Model file for the job. Use its own axes, mm. Coordinates: 2 decimals unless noted, no trailing zeros. Loops run counter-clockwise (first coordinate to the right, second up) from the corner with the lowest first, then second, coordinate; pieces in that order, holes last. Notation, with made-up numbers: M -24,70.5 L 34,70.5 A30 ccw 34,101.5 Z; hole C 45,71.5 d11. An arc over 180 degrees is marked long. One line per question, with ' | ' between items. Start each with the question number.
Autodesk Inventor part; units mm, degrees
ref_plane "YZ Plane" through (0, 0, 0) normal (1, 0, 0) x (0, 1, 0)
ref_plane "XZ Plane" through (0, 0, 0) normal (0, 1, 0) x (-1, 0, 0)
ref_plane "XY Plane" through (0, 0, 0) normal (0, 0, 1) x (1, 0, 0)
sketch "Sketch1" plane through (0, 0, 0) normal (0, 0, 1) x (1, 0, 0)
  circle A0 centre (0, 0) radius 8
  line L0 (3.3198, 5.75) -> (6.6395, 0)
  line L1 (6.6395, 0) -> (3.3198, -5.75)
  line L2 (3.3198, -5.75) -> (-3.3198, -5.75)
  line L3 (-3.3198, -5.75) -> (-6.6395, 0)
  line L4 (-6.6395, 0) -> (-3.3198, 5.75)
  line L5 (-3.3198, 5.75) -> (3.3198, 5.75)
  circle A1 centre (0, 0) radius 3.2
  dimension "d0" = 16
  dimension "d1" = 11.5
  dimension "d2" = 6.4
extrude "Extrusion1" add sketch "Sketch1" along normal blind 17 contours A0 | L0 L1 L2 L3 L4 L5 | A1
fillet "Fillet1" radius 8 1 edges at (-8, 0, 17)
extrude "Extrusion2" cut sketch "Sketch1" along normal blind 13.5 contours A1
extrude "Extrusion3" cut sketch "Sketch1" along normal blind 5.8 contours L0 L1 L2 L3 L4 L5
properties part number "BreakerBoltCover"
(1) Two-plate mould, pull along Y, no slides. Class faces 1 (the face through (1, -6, 0)), 2 (the face through (-1.73, 7.81, 4.44)), 3 (the face through (-5.003, 2.835, 2.859)): pulls with the +Y half, pulls with the -Y half, needs draft (parallel to the pull), parting line crosses it, or undercut.
(2) Band-saw the part on A-A on z = 5. Write the cut outline in (x, y), then the cut area to 3 significant figures.
(3) Pin check, flat tips, straight feed: P1, Ø3.5, axis at x = 1, y = -1.5, coming from the -Z side; P2, Ø2, axis at y = 5.5, z = 2.5, coming from the -X side; P3, Ø6, axis at x = -4.5, z = 12, coming from the +Y side. Stop position of each tip, or through.
(4) Band-saw the part on C-C on y = 4.25. Write the cut outline in (x, z), then the cut area to 3 significant figures.
(5) Band-saw the part on D-D on z = 8.25. Write the cut outline in (x, y), then the cut area to 3 significant figures.
(6) Band-saw the part on B-B on x = 0. Write the cut outline in (y, z), then the cut area to 3 significant figures.
(7) Drill centre lines: line 1 (Y direction, x = 0, z = 9); line 2 (Y direction, x = 0.75, z = 5); line 3 (X direction, y = -2.5, z = 12.5). Where is each one in solid material? Low to high. Write a range as [from, to].
Computed values:
1) face 1: needs draft | face 2: parting line crosses it | face 3: undercut
2) outline: C 0,0 d16; hole M -6.64,0 L -3.32,-5.75 L 3.32,-5.75 L 6.64,0 L 3.32,5.75 L -3.32,5.75 Z | area: 86.5 mm^2
3) P1: z = 5.8 | P2: x = -6.61 | P3: y = 7.63
4) outline: M -6.78,0 L -4.19,0 L -4.19,5.8 L 4.19,5.8 L 4.19,0 L 6.78,0 L 6.78,9 A6.78 ccw -6.78,9 Z | area: 146 mm^2
5) outline: C 0,0 d16; hole C 0,0 d6.4 | area: 169 mm^2
6) outline: M -8,0 L -5.75,0 L -5.75,5.8 L -3.2,5.8 L -3.2,13.5 L 3.2,13.5 L 3.2,5.8 L 5.75,5.8 L 5.75,0 L 8,0 L 8,9 A8 ccw -8,9 Z | area: 129 mm^2
7) line 1: [-8, -3.2], [3.2, 8] | line 2: [-7.96, -5.75], [5.75, 7.96] | line 3: [-6.75, -2], [2, 6.75]
